from build123d import *
from OCP.BRepFilletAPI import BRepFilletAPI_MakeChamfer

# Parameters (mm, degrees)
SKETCH_1_W          = 20.2
SKETCH_1_H          = 7.2
EXTRUDE_1_DEPTH     = 10
SKETCH_2_W          = 0.5
SKETCH_2_H          = 3.5
EXTRUDE_2_DEPTH     = 4
CUT_EXTRUDE_1_REACH = 23.64
SKETCH_3_R          = 0.75
CHAMFER_1_SIZE      = 1
CHAMFER_1_SIZE2     = 0.700207538
SKETCH_4_R          = 1
CUT_EXTRUDE_2_DEPTH = 16.932670837
SKETCH_5_W          = 2
SKETCH_5_H          = 4
EXTRUDE_3_DEPTH     = 1
FILLET_1_R          = 0.6


with BuildPart() as part:
    # Эскиз1 → Бобышка-Вытянуть1 (new body)
    with BuildSketch(Plane(origin=(0, 0, 0), x_dir=(1, 0, 0), z_dir=(0, 1, 0))):
        Rectangle(SKETCH_1_W, SKETCH_1_H)
    extrude(amount=EXTRUDE_1_DEPTH)

    # Эскиз2 → Бобышка-Вытянуть2 (add)
    with BuildSketch(Plane(origin=(0, 0, 0), x_dir=(-1, 0, 0), z_dir=(0, -1, 0))):
        with Locations((-7, 0)):
            Rectangle(SKETCH_2_W, SKETCH_2_H)
        Rectangle(SKETCH_2_W, SKETCH_2_H)
        with Locations((8.5, 0)):
            Rectangle(SKETCH_2_W, SKETCH_2_H)
    extrude(amount=EXTRUDE_2_DEPTH)

    # Вырез-Вытянуть1: up to this face of the body (flat: up to its plane)
    cut_extrude_1_end = Plane(part.part.faces().sort_by_distance((7.25, -2, 0))[0])
    # Эскиз3 → Вырез-Вытянуть1 (cut, up to the picked face)
    with BuildSketch(Plane.ZY.offset(8.75), mode=Mode.PRIVATE) as cut_extrude_1_sk1:
        with Locations((0, -2.680856865)):
            Circle(SKETCH_3_R)
    cut_extrude_1_tool1 = split(extrude(cut_extrude_1_sk1.sketch, amount=-CUT_EXTRUDE_1_REACH, mode=Mode.PRIVATE), bisect_by=cut_extrude_1_end, keep=Keep.BOTH, mode=Mode.PRIVATE)
    add(cut_extrude_1_tool1.solids().sort_by(Axis((-8.75, -2.680857, 0), (1, 0, 0)))[0], mode=Mode.SUBTRACT)

    # Фаска1: one chamfer whose edges measure the first distance from different faces: ONE call of the kernel's chamfer builder (chamfer() names one face for all edges)
    chamfer_1_edges_1 = [part.edges().sort_by_distance(p)[0] for p in [
        (0, -4, 1.75),
    ]]
    chamfer_1_side_1 = [part.faces().sort_by_distance(p)[0] for p in [
        (0, -2, 1.75),
    ]]
    chamfer_1_edges_2 = [part.edges().sort_by_distance(p)[0] for p in [
        (0, -4, -1.75),
    ]]
    chamfer_1_side_2 = [part.faces().sort_by_distance(p)[0] for p in [
        (0, -2, -1.75),
    ]]
    chamfer_1_edges_3 = [part.edges().sort_by_distance(p)[0] for p in [
        (7, -4, -1.75),
    ]]
    chamfer_1_side_3 = [part.faces().sort_by_distance(p)[0] for p in [
        (7, -2, -1.75),
    ]]
    chamfer_1_edges_4 = [part.edges().sort_by_distance(p)[0] for p in [
        (7, -4, 1.75),
    ]]
    chamfer_1_side_4 = [part.faces().sort_by_distance(p)[0] for p in [
        (7, -2, 1.75),
    ]]
    chamfer_1_edges_5 = [part.edges().sort_by_distance(p)[0] for p in [
        (-8.5, -4, -1.75),
    ]]
    chamfer_1_side_5 = [part.faces().sort_by_distance(p)[0] for p in [
        (-8.5, -2, -1.75),
    ]]
    chamfer_1_edges_6 = [part.edges().sort_by_distance(p)[0] for p in [
        (-8.5, -4, 1.75),
    ]]
    chamfer_1_side_6 = [part.faces().sort_by_distance(p)[0] for p in [
        (-8.5, -2, 1.75),
    ]]
    chamfer_1 = BRepFilletAPI_MakeChamfer(part.part.solid().wrapped)
    for e in chamfer_1_edges_1:
        chamfer_1.Add(CHAMFER_1_SIZE, CHAMFER_1_SIZE2, e.wrapped, chamfer_1_side_1[0].wrapped)  # the first distance lies on this face
    for e in chamfer_1_edges_2:
        chamfer_1.Add(CHAMFER_1_SIZE, CHAMFER_1_SIZE2, e.wrapped, chamfer_1_side_2[0].wrapped)  # the first distance lies on this face
    for e in chamfer_1_edges_3:
        chamfer_1.Add(CHAMFER_1_SIZE, CHAMFER_1_SIZE2, e.wrapped, chamfer_1_side_3[0].wrapped)  # the first distance lies on this face
    for e in chamfer_1_edges_4:
        chamfer_1.Add(CHAMFER_1_SIZE, CHAMFER_1_SIZE2, e.wrapped, chamfer_1_side_4[0].wrapped)  # the first distance lies on this face
    for e in chamfer_1_edges_5:
        chamfer_1.Add(CHAMFER_1_SIZE, CHAMFER_1_SIZE2, e.wrapped, chamfer_1_side_5[0].wrapped)  # the first distance lies on this face
    for e in chamfer_1_edges_6:
        chamfer_1.Add(CHAMFER_1_SIZE, CHAMFER_1_SIZE2, e.wrapped, chamfer_1_side_6[0].wrapped)  # the first distance lies on this face
    add(Compound.cast(chamfer_1.Shape()), mode=Mode.REPLACE)

    # Эскиз4 → Вырез-Вытянуть2 (cut, through all)
    with BuildSketch(Plane(origin=(0, 0, -3.6), x_dir=(-1, 0, 0), z_dir=(0, 0, -1))):
        with Locations((-5.1, 2)):
            Circle(SKETCH_4_R)
        with Locations(Location((5.1, 2, 0), (0, 0, 180))):
            Circle(SKETCH_4_R)
    extrude(amount=-CUT_EXTRUDE_2_DEPTH, mode=Mode.SUBTRACT)

    # Эскиз5 → Бобышка-Вытянуть3 (add)
    with BuildSketch(Plane(origin=(0, 10, 0), x_dir=(1, 0, 0), z_dir=(0, 1, 0))):
        with Locations((-2.1, -0.1)):
            Rectangle(SKETCH_5_W, SKETCH_5_H)
    extrude(amount=EXTRUDE_3_DEPTH)

    # Скругление1
    fillet_1_edges = [part.edges().sort_by_distance(p)[0] for p in [
        (-3.1, 11, 0.1),
        (-1.1, 11, 0.1),
    ]]
    fillet(fillet_1_edges, radius=FILLET_1_R)


solid = part.part
Input: part model. Units: mm. Frame: model coordinates. A direction names the side the tool comes from. Round coordinates to 2 decimals unless told otherwise and drop trailing zeros. Order: outer loops, then holes, each group sorted by start corner. A loop starts at its lowest first (then second) coordinate and runs counter-clockwise, first axis right, second up.
1. Cut plane A-A, the plane x = -5.1. Output: boundary loops of the cut face in (y, z), then the cut area to 3 significant figures.
The answers:
outline: (0, -3.6) - (1, -3.6) - (1, 3.6) - (0, 3.6) - close; (3, -3.6) - (10, -3.6) - (10, 3.6) - (3, 3.6) - close
area: 57.6 mm2
2. Cut plane B-B, the plane y = -0.25. Output: boundary loops of the cut face in (x, z).
The answers:
outline: (-8.75, -1.75) - (-8.25, -1.75) - (-8.25, 1.75) - (-8.75, 1.75) - close; (-0.25, -1.75) - (0.25, -1.75) - (0.25, 1.75) - (-0.25, 1.75) - close; (6.75, -1.75) - (7.25, -1.75) - (7.25, 1.75) - (6.75, 1.75) - close
3. Cut plane D-D, the plane y = 2. Output: boundary loops of the cut face in (x, z).
The answers:
outline: (-10.1, -3.6) - (-6.1, -3.6) - (-6.1, 3.6) - (-10.1, 3.6) - close; (-4.1, -3.6) - (4.1, -3.6) - (4.1, 3.6) - (-4.1, 3.6) - close; (6.1, -3.6) - (10.1, -3.6) - (10.1, 3.6) - (6.1, 3.6) - close
4. Pin query (flat end, axial travel): P1, Ø3, axis at x = 6, y = -2, coming from the -Z side; P2, Ø3, axis at y = -2.5, z = -1, coming from the -X side; P3, Ø1.4, axis at y = -2.68, z = 0, coming from the -X side; P4, Ø3, axis at x = -5.1, y = 2, coming from the +Z side. Return the tip coordinate at first contact, or that it passes through.
The answers:
P1: stops at z = -1.75
P2: stops at x = -8.75
P3: passes through
P4: stops at z = 3.6
5. Set-up query: faces 5 (the face through (-8.75, -1.5, 0)), 6 (the face through (-2.1, 10.5, 2.1)), 7 (the face through (-0.25, -1.5, 0)), 8 (the face through (7.25, -1.5, 0)). Return all of +Z, -Z, +X, -X, +Y, -Y with unobstructed straight access to the full face (end or side cutting, diameter ignored); none if empty.
The answers:
face 5: +Z, -Z, -X, -Y
face 6: +Z, +X, -X, +Y
face 7: +Z, -Z, -Y
face 8: +Z, -Z, +X, -Y
6. Cut plane C-C, the plane z = 0. State how many separate pieces and enclosed holes the cut face has, then the cut area to 3 significant figures.
The answers:
separate pieces: 4
enclosed holes: 2
area: 201 mm2
7. Material intervals for line 1 (Y direction, x = 7.05, z = 0); line 2 (Y direction, x = -5, z = -0.75); line 3 (X direction, y = 2.5, z = 2), sorted ascending.
The answers:
line 1: y = -4 to -3.43, -1.93 to 10
line 2: y = 0 to 1.01, 2.99 to 10
line 3: x = -10.1 to -5.97, -4.23 to 4.23, 5.97 to 10.1
8. Mould query, pull axis Z, two halves, no side actions, for faces 1 (the face through (-8.504, -3.413, -0.163)), 2 (the face through (-2.1, 10.5, -1.9)), 3 (the face through (6.996, -3.413, -0.163)), 4 (the face through (0.25, -1.5, 0)). Classes: released by +Z, released by -Z, zero draft, split by the parting line, or undercut.
The answers:
face 1: undercut
face 2: released by -Z
face 3: undercut
face 4: zero draft
